```python
from build123d import *

# Parameters (mm, degrees)
SKETCH1_R           = 14.9
SKETCH1_R_2         = 1.6
BOSS_EXTRUDE1_DEPTH = 3.5
SKETCH2_R           = 1.5
BOSS_EXTRUDE2_DEPTH = 2
FILLET1_R           = 0.3
SKETCH3_R           = 17
SKETCH3_R_2         = 1.6
BOSS_EXTRUDE3_DEPTH = 5.5
BOSS_EXTRUDE4_DEPTH = 3
FILLET2_R           = 0.5


with BuildPart() as part:
    # Sketch1 → Boss-Extrude1 (new body)
    with BuildSketch(Plane(origin=(0, 0, 0), x_dir=(1, 0, 0), z_dir=(0, 1, 0))):
        Circle(SKETCH1_R)
        with Locations((0, 12)):
            Circle(SKETCH1_R_2, mode=Mode.SUBTRACT)
        with Locations((12, 0)):
            Circle(SKETCH1_R_2, mode=Mode.SUBTRACT)
        with Locations((0, -12)):
            Circle(SKETCH1_R_2, mode=Mode.SUBTRACT)
        with Locations((-12, 0)):
            Circle(SKETCH1_R_2, mode=Mode.SUBTRACT)
    extrude(amount=BOSS_EXTRUDE1_DEPTH)

    # Sketch2 → Boss-Extrude2 (add)
    with BuildSketch(Plane.XZ):
        with Locations((3.5, -3.5)):
            Circle(SKETCH2_R)
        with Locations((-3.5, 3.5)):
            Circle(SKETCH2_R)
    extrude(amount=BOSS_EXTRUDE2_DEPTH)

    # Fillet1
    fillet1_edges = [part.edges().sort_by_distance(p)[0] for p in [
        (2, -2, -3.5),
        (-5, -2, 3.5),
    ]]
    fillet(fillet1_edges, radius=FILLET1_R)

    # Sketch3 → Boss-Extrude3 (add)
    with BuildSketch(Plane(origin=(0, 3.5, 0), x_dir=(1, 0, 0), z_dir=(0, 1, 0))):
        Circle(SKETCH3_R)
        with Locations((12, 0)):
            Circle(SKETCH3_R_2, mode=Mode.SUBTRACT)
        with Locations((0, -12)):
            Circle(SKETCH3_R_2, mode=Mode.SUBTRACT)
        with Locations((-12, 0)):
            Circle(SKETCH3_R_2, mode=Mode.SUBTRACT)
        with Locations((0, 12)):
            Circle(SKETCH3_R_2, mode=Mode.SUBTRACT)
    extrude(amount=BOSS_EXTRUDE3_DEPTH)

    # Sketch4 → Boss-Extrude4 (add)
    with BuildSketch(Plane(origin=(0, 9, 0), x_dir=(1, 0, 0), z_dir=(0, 1, 0))):
        with BuildLine():
            Line((-4.101219331, 1.414213562), (-1.414213562, 4.101219331))
            ThreePointArc((-1.414213562, 4.101219331), (0, 4.687005769), (1.414213562, 4.101219331))
            Line((1.414213562, 4.101219331), (4.101219331, 1.414213562))
            ThreePointArc((4.101219331, 1.414213562), (4.687005769, 0), (4.101219331, -1.414213562))
            Line((4.101219331, -1.414213562), (1.414213562, -4.101219331))
            ThreePointArc((1.414213562, -4.101219331), (0, -4.687005769), (-1.414213562, -4.101219331))
            Line((-1.414213562, -4.101219331), (-4.101219331, -1.414213562))
            ThreePointArc((-4.101219331, -1.414213562), (-4.687005769, 0), (-4.101219331, 1.414213562))
        make_face()
    extrude(amount=BOSS_EXTRUDE4_DEPTH)

    # Fillet2
    fillet2_edges = [part.edges().sort_by_distance(p)[0] for p in [
        (4.687005769, 12, 0),
        (2.757716447, 12, -2.757716447),
        (0, 12, -4.687005769),
        (-2.757716447, 12, -2.757716447),
        (-4.687005769, 12, 0),
        (-2.757716447, 12, 2.757716447),
        (0, 12, 4.687005769),
        (2.757716447, 12, 2.757716447),
    ]]
    fillet(fillet2_edges, radius=FILLET2_R)


solid = part.part
```
Build history of the part. All positions in model axes, mm. A direction names the side the tool comes from. Give positions to 0.01 mm unless a question says otherwise; leave off trailing zeros. Order: outer loops, then holes, each group sorted by start corner. A loop starts at its lowest first (then second) coordinate and runs counter-clockwise, first axis right, second up. Notation, with made-up numbers: M 47.5,33 L 91.5,33 A19 cw 91.5,65 Z; hole C 16.5,11 d8. An arc over 180 degrees is marked long. Return JSON: item names as keys, results as strings.
Q1. Band-saw the part on D-D (x = 12.5). Give the cut face in (y, z).
Answer list:
{"outline": "M 0,-8.11 L 3.5,-8.11 L 3.5,-11.52 L 9,-11.52 L 9,-1.52 L 0,-1.52 Z; M 0,1.52 L 9,1.52 L 9,11.52 L 3.5,11.52 L 3.5,8.11 L 0,8.11 Z"}
Q2. Band-saw the part on B-B (z = 0). Give the cut face in (x, y), then the cut area to 3 significant figures.
Answer list:
{"outline": "M -17,3.5 L -14.9,3.5 L -14.9,0 L -13.6,0 L -13.6,9 L -17,9 Z; M -10.4,0 L 10.4,0 L 10.4,9 L 4.69,9 L 4.69,11.5 A0.5 ccw 4.19,12 L -4.19,12 A0.5 ccw -4.69,11.5 L -4.69,9 L -10.4,9 Z; M 13.6,0 L 14.9,0 L 14.9,3.5 L 17,3.5 L 17,9 L 13.6,9 Z", "area": "262 mm^2"}
Q3. Wall check: probe 1 along X at (y, z) = (5, 0); probe 2 along X at (y, z) = (2.5, 0); probe 3 along Y at (x, z) = (-9, 13.5). Give the ranges that are in metal, low to high. Write a range as from..to.
Answer list:
{"probe 1": "x = -17..-13.6, -10.4..10.4, 13.6..17", "probe 2": "x = -14.9..-13.6, -10.4..10.4, 13.6..14.9", "probe 3": "y = 3.5..9"}
Q4. Flat gauge pins, fed straight in: pin 1 (3 mm diameter, centred on y = 9, z = 4.5, fed in from -X); pin 2 (1 mm diameter, centred on y = 1.5, z = 13, fed in from -X); pin 3 (5 mm diameter, centred on x = 12, z = 0, fed in from -Y). Where does each tip first touch, or does it go through?
Answer list:
{"pin 1": "stops at x = -16.73", "pin 2": "stops at x = -8.11", "pin 3": "stops at y = 0"}
Q5. 3-axis set-ups, long thin cutter, end or side, ignore diameter. For faces 5 (the face through (4.687, 10.232, -0.022)), 6 (the face through (-2.739, 10.232, 2.777)), 7 (the face through (-0.022, 10.232, -4.687)), 8 (the face through (-2.07, -0.84, 3.95)): which of +Z, -Z, +X, -X, +Y, -Y reach the whole face in a straight line?
Answer list:
{"face 5": "+X, +Y", "face 6": "+Z, -X, +Y", "face 7": "-Z, +Y", "face 8": "-Y"}
Q6. Two-plate mould, pull along X, no slides. Class faces 1 (the face through (-0.35, 4.44, 13.56)), 2 (the face through (10.4, 4.44, -0.07)), 3 (the face through (-2.638, 11.85, -2.676)), 4 (the face through (2.739, 10.232, -2.777)): pulls with the +X half, pulls with the -X half, needs draft (parallel to the pull), parting line crosses it, or undercut.
Answer list:
{"face 1": "undercut", "face 2": "undercut", "face 3": "pulls with the -X half", "face 4": "pulls with the +X half"}
Q7. Band-saw the part on C-C (y = 8.25). Give the cut face in (x, z), then the cut area to 3 significant figures.
Answer list:
{"outline": "C 0,0 d34; hole C -12,0 d3.2; hole C 0,-12 d3.2; hole C 0,12 d3.2; hole C 12,0 d3.2", "area": "876 mm^2"}
Q8. Band-saw the part on A-A (x = 0). Give the cut face in (y, z).
Answer list:
{"outline": "M 0,-14.9 L 3.5,-14.9 L 3.5,-17 L 9,-17 L 9,-13.6 L 0,-13.6 Z; M 0,-10.4 L 9,-10.4 L 9,-4.69 L 11.5,-4.69 A0.5 ccw 12,-4.19 L 12,4.19 A0.5 ccw 11.5,4.69 L 9,4.69 L 9,10.4 L 0,10.4 Z; M 0,13.6 L 9,13.6 L 9,17 L 3.5,17 L 3.5,14.9 L 0,14.9 Z"}
